Autodesk Fusion 360 part; units mm, degrees
sketch "Sketch2" plane through (0, 0, 0) normal (0, 1, 0) x (1, 0, 0)
  line L0 (-30, 0) -> (-30, 90)
  line L1 (30, 100) -> (30, 150)
  line L2 (30, 150) -> (90, 150)
  line L3 (30, 150) -> (-90, 150)
  line L4 (-90, 100) -> (-40, 100)
  arc A0 (-30, 90) -> (-40, 100) centre (-40, 90) ccw
  line L5 (40, 100) -> (90, 100)
  arc A1 (-30, 0) -> (30, 0) centre (0, 0) ccw
  arc A2 (30, 0) -> (-30, 0) centre (0, 0) ccw
  arc A3 (-15, 0) -> (15, 0) centre (0, 0) ccw
  arc A4 (15, 0) -> (-15, 0) centre (0, 0) ccw
  line L6 (30, 0) -> (30, 90)
  arc A5 (90, 100) -> (90, 150) centre (90, 125) ccw
  arc A6 (-90, 150) -> (-90, 100) centre (-90, 125) ccw
  arc A7 (40, 100) -> (30, 90) centre (40, 90) ccw
  circle A8 centre (-90, 125) radius 10
  circle A9 centre (90, 125) radius 10
  point P0 (-30, 150)
  dimension "d1" = 150
  dimension "d2" = 60
  dimension "d3" = 60
  dimension "d4" = 120
  dimension "d5" = 30
  dimension "d6" = 25
  dimension "d7" = 25
  dimension "d8" = 25
  dimension "d9" = 10
  dimension "d10" = 10
  dimension "d11" = 20
  dimension "d12" = 20
extrude "Extrude1" add sketch "Sketch2" along normal blind 40 contours A1 A2
extrude "Extrude2" add sketch "Sketch2" along normal blind 30 contours L0 L2 L3 L4 A0 L5 A2 L6 A5 A6 A7
sketch "Sketch3" plane through (0, 30, 0) normal (0, 1, 0) x (-1, 0, 0)
  circle A0 centre (-90, -125) radius 10
  circle A1 centre (90, -125) radius 10
  arc A2 (-90, -100) -> (-90, -150) centre (-90, -125) ccw
  line L0 (-90, -150) -> (90, -150)
  arc A3 (90, -150) -> (90, -100) centre (90, -125) ccw
  line L1 (90, -100) -> (40, -100)
  arc A4 (30, -90) -> (40, -100) centre (40, -90) ccw
  line L2 (30, -90) -> (30, 0)
  arc A5 (-30, 0) -> (30, 0) centre (0, 0) ccw
  line L3 (-30, 0) -> (-30, -90)
  arc A6 (-40, -100) -> (-30, -90) centre (-40, -90) ccw
  line L4 (-40, -100) -> (-90, -100)
sketch "Sketch4" plane through (30, 0, 0) normal (1, 0, 0) x (0, 1, 0)
  line L0 (0, 0) -> (0, -90)
  line L1 (0, -90) -> (30, -90)
  line L2 (30, -90) -> (30, 0)
  line L3 (30, 0) -> (0, 0)
  line L4 (30, -150) -> (30, -70)
  line L5 (105, -84.5349) -> (105, -85)
  arc A0 (109.7565, -134.5434) -> (109.7565, -85.4566) centre (105, -110) ccw
  arc A1 (105, -122.5) -> (105, -97.5) centre (105, -110) ccw
  arc A2 (105, -97.5) -> (105, -122.5) centre (105, -110) ccw
  line L6 (30, -70) -> (109.7565, -85.4566)
  line L7 (30, -150) -> (109.7565, -134.5434)
  dimension "d17" = 80
  dimension "d20" = 25
  dimension "d24" = 0
  dimension "d25" = 0
extrude "Extrude3" add sketch "Sketch4" against normal blind 15 contours L2 L4 A0 L6 L7
sketch "Sketch7" plane through (-30, 0, 0) normal (-1, 0, 0) x (0, -1, 0)
  line L0 (0, -90) -> (0, 0)
  line L1 (0, 0) -> (-30, 0)
  line L2 (-30, 0) -> (-30, -90)
  line L3 (-30, -90) -> (0, -90)
  line L4 (-30, -70) -> (-30, -150)
  circle A0 centre (-105, -110) radius 12.5
  line L5 (-105, -84.5349) -> (-109.7565, -85.4566)
  line L6 (-105, -135.4651) -> (-109.7565, -134.5434)
  line L7 (-30, -150) -> (-105, -135.4651)
  line L8 (-30, -70) -> (-105, -84.5349)
  arc A1 (-109.7565, -85.4566) -> (-109.7565, -134.5434) centre (-105, -110) ccw
  dimension "d29" = 25
extrude "Extrude4" add sketch "Sketch7" against normal blind 15 contours L2 L4 L5 L6 L7 L8 A1
CAD build for the part. Positions are in the model's coordinates, mm. A direction names the side the tool comes from. Round coordinates to 2 decimals unless told otherwise and drop trailing zeros. Order: outer loops, then holes, each group sorted by start corner. A loop starts at its lowest first (then second) coordinate and runs counter-clockwise, first axis right, second up. Notation, with made-up numbers: (42, -21) -> (81, -21) arc R37 ccw to (81, 18) -> close; hole circle Ø8 at (60.5, 30). An arc over 180 degrees is marked (long way). One line per question, with ' | ' between items.
Q1. Slice it at A-A (x = 0). Write the cut outline in (y, z).
Completed:
outline: (0, -150) -> (30, -150) -> (30, -30) -> (40, -30) -> (40, -15) -> (0, -15) -> close; (0, 15) -> (40, 15) -> (40, 30) -> (0, 30) -> close
Q2. Slice it at B-B (y = 12.5). Write the cut outline in (x, z), then the cut area to 3 significant figures.
Completed:
outline: (-90, -150) -> (90, -150) arc R25 ccw to (90, -100) -> (40, -100) arc R10 cw to (30, -90) -> (30, 0) arc R30 ccw to (-30, 0) -> (-30, -90) arc R10 cw to (-40, -100) -> (-90, -100) arc R25 ccw to start; hole circle Ø20 at (-90, -125); hole circle Ø30 at (0, 0); hole circle Ø20 at (90, -125) | area: 17,100 mm^2
Q3. Which spindle directions (+Z, -Z, +X, -X, +Y, -Y) get a long thin tool onto all of the face, cutting with end or side? Do faces 1 (the flat face through (-73, 30, -127)), 2 (the flat face through (-65, 15, -100)), 3 (the flat face through (72, 30, -127)), 4 (the flat face through (-30, 51, -91)). Say none if no direction does.
Completed:
face 1: +Z, -Z, -X, +Y | face 2: +Z, -X, +Y, -Y | face 3: +Z, -Z, +X, +Y | face 4: +Z, -X, +Y
Q4. Slice it at C-C (z = 4.5). Write the cut outline in (x, y).
Completed:
outline: (-29.66, 0) -> (-14.31, 0) -> (-14.31, 40) -> (-29.66, 40) -> close; (14.31, 0) -> (29.66, 0) -> (29.66, 40) -> (14.31, 40) -> close
Q5. Drop flat-ended pins along their axis: pin 1 (6 mm diameter, centred on x = -38, y = 15, fed in from +Z); pin 2 (10 mm diameter, centred on x = 26, y = 97, fed in from +Z); pin 3 (9 mm diameter, centred on x = 69, y = 16, fed in from +Z). Give the stop position or say it passes through.
Completed:
pin 1: stops at z = -98.66 | pin 2: stops at z = -82.02 | pin 3: stops at z = -100
Q6. Two-plate mould, pull along Z, no slides. Class faces 5 (the flat face through (6, 40, -14)), 6 (the cylindrical face through (114.994, 14.79, -125.55)), 7 (the flat face through (0, 30, -76)), 8 (the cylindrical face through (82.63, 14.79, -118.24)): released by +Z, released by -Z, zero draft, split by the parting line, or undercut.
Completed:
face 5: zero draft | face 6: split by the parting line | face 7: undercut | face 8: undercut
Q7. Probe probe 1 along Z at (x, y) = (90, 12.25); probe 2 along X at (y, z) = (75, -95); probe 3 along X at (y, z) = (10, -125). List the from-to ranges inside material, lowest first.
Completed:
probe 1: z = -150 to -135, -115 to -100 | probe 2: x = -30 to -15, 15 to 30 | probe 3: x = -115 to -100, -80 to 80, 100 to 115
Q8. Slice it at D-D (z = -118). Write the cut outline in (x, y), then the cut area to 3 significant figures.
Completed:
outline: (-114, 0) -> (-97.14, 0) -> (-97.14, 30) -> (-114, 30) -> close; (-82.86, 0) -> (82.86, 0) -> (82.86, 30) -> (30, 30) -> (30, 95.4) -> (15, 95.4) -> (15, 30) -> (-15, 30) -> (-15, 95.4) -> (-30, 95.4) -> (-30, 30) -> (-82.86, 30) -> close; (-30, 114.6) -> (-15, 114.6) -> (-15, 128.69) -> (-30, 128.69) -> close; (15, 114.6) -> (30, 114.6) -> (30, 128.69) -> (15, 128.69) -> close; (97.14, 0) -> (114, 0) -> (114, 30) -> (97.14, 30) -> close | area: 8,370 mm^2
